from build123d import *

# Parameters (mm, degrees)
SKETCH_1_R               = 5
SKETCH_1_R_2             = 2.15
EXTRUDE_1_DEPTH          = 3
SKETCH_2_R               = 1.5
CUT_EXTRUDE_1_DEPTH      = 117.657618697
CUT_EXTRUDE_3_DEPTH      = 117.657618697
SKETCH_5_W               = 40
SKETCH_5_H               = 20
SKETCH_5_R               = 2.15
EXTRUDE_2_DEPTH          = 3
SKETCH_6_R               = 5
CUT_EXTRUDE_4_DEPTH      = 117.657618697
SKETCH_7_R               = 1.5
EXTRUDE_4_DEPTH          = 3
CUT_EXTRUDE_6_DEPTH      = 117.657618697
CUT_EXTRUDE_6_DEPTH_BACK = 117.657618697
SKETCH_9_R               = 1.6
CUT_EXTRUDE_7_DEPTH      = 117.657618697
SKETCH_10_W              = 79.9
SKETCH_10_H              = 10
SKETCH_10_R              = 1.6
EXTRUDE_5_DEPTH          = 3
FILLET_1_R               = 2.5


with BuildPart() as part:
    # ｽｹｯﾁ1 → ﾎﾞｽ - 押し出し1 (new body)
    with BuildSketch(Plane.XY):
        Polygon((10, 60), (0, 60), (0, 0), (100, 0), (100, 50), (100, 60), (50, 60), (50, 40), (10, 40), align=None)
        with Locations((20, 20)):
            Circle(SKETCH_1_R, mode=Mode.SUBTRACT)
        with Locations((5.25, 45)):
            Circle(SKETCH_1_R_2, mode=Mode.SUBTRACT)
        with Locations((5.25, 55)):
            Circle(SKETCH_1_R_2, mode=Mode.SUBTRACT)
        with Locations((54.75, 45)):
            Circle(SKETCH_1_R_2, mode=Mode.SUBTRACT)
        with Locations((54.75, 55)):
            Circle(SKETCH_1_R_2, mode=Mode.SUBTRACT)
    extrude(amount=EXTRUDE_1_DEPTH)

    # ｽｹｯﾁ2 → ｶｯﾄ - 押し出し1 (cut, through all)
    with BuildSketch(Plane.XY.offset(3)):
        with Locations((95, 35)):
            Circle(SKETCH_2_R)
    extrude(amount=-CUT_EXTRUDE_1_DEPTH, mode=Mode.SUBTRACT)

    # ｽｹｯﾁ4 → ｶｯﾄ - 押し出し3 (cut, through all)
    with BuildSketch(Plane.XY.offset(3)):
        with BuildLine():
            ThreePointArc((30.606601718, 9.393398282), (11.666446505, 7.527955815), (6.141807012, 25.740251485))
            ThreePointArc((6.141807012, 25.740251485), (5.992593584, 34.011854082), (1.731818145, 41.103219734))
            ThreePointArc((1.731818145, 41.103219734), (1.633577382, 41.194216579), (1.537689399, 41.287689399))
            ThreePointArc((1.537689399, 41.287689399), (0.399632454, 42.99091198), (0, 45))
            Line((0, 45), (0, 0))
            Line((0, 0), (100, 0))
            Line((100, 0), (100, 35))
            ThreePointArc((100, 35), (98.535533906, 31.464466094), (95, 30))
            ThreePointArc((95, 30), (93.906844507, 30.120962075), (92.866581158, 30.477995572))
            ThreePointArc((92.866581158, 30.477995572), (59.698938801, 28.658859349), (31.76111788, 10.689999666))
            ThreePointArc((31.76111788, 10.689999666), (31.202634234, 10.024981894), (30.606601718, 9.393398282))
        make_face()
    extrude(amount=-CUT_EXTRUDE_3_DEPTH, mode=Mode.SUBTRACT)

    # ｽｹｯﾁ5 → ﾎﾞｽ - 押し出し2 (add, through all)
    with BuildSketch(Plane.XY.offset(3)):
        with Locations((30, 50)):
            Rectangle(SKETCH_5_W, SKETCH_5_H)
        with Locations((5.25, 55)):
            Circle(SKETCH_5_R)
        with Locations((5.25, 45)):
            Circle(SKETCH_5_R)
        with Locations((54.75, 45)):
            Circle(SKETCH_5_R)
        with Locations((54.75, 55)):
            Circle(SKETCH_5_R)
    extrude(amount=-EXTRUDE_2_DEPTH)

    # ｽｹｯﾁ6 → ｶｯﾄ - 押し出し4 (cut, through all)
    with BuildSketch(Plane.XY.offset(3)):
        with Locations((20, 50)):
            Circle(SKETCH_6_R)
    extrude(amount=-CUT_EXTRUDE_4_DEPTH, mode=Mode.SUBTRACT)

    # ｽｹｯﾁ7 → ﾎﾞｽ - 押し出し4 (add, through all)
    # profile 1 of 2: a face of its own
    with BuildSketch(Plane.XY.offset(3)):
        with BuildLine():
            ThreePointArc((0, 45), (-1.007160055, 41.702552665), (-3.074339462, 38.943150628))
            ThreePointArc((-3.074339462, 38.943150628), (2.194117441, 39.492866419), (5, 35))
            ThreePointArc((5, 35), (2.338239569, 30.580425844), (-2.813054288, 30.866390733))
            ThreePointArc((-2.813054288, 30.866390733), (2.156646174, 25.048507639), (5.133931253, 18))
            ThreePointArc((5.133931253, 18), (5.125569714, 21.936833416), (6.141807012, 25.740251485))
            ThreePointArc((6.141807012, 25.740251485), (5.992593584, 34.011854082), (1.731818145, 41.103219734))
            ThreePointArc((1.731818145, 41.103219734), (0.4524509, 42.867859613), (0, 45))
        make_face()
    # profile 2 of 2: a face of its own
    with BuildSketch(Plane.XY.offset(3)):
        with BuildLine():
            ThreePointArc((-3.074339462, 38.943150628), (-3.301799792, 38.735793058), (-3.535533906, 38.535533906))
            ThreePointArc((-3.535533906, 38.535533906), (-5, 35), (-3.535533906, 31.464466094))
            ThreePointArc((-3.535533906, 31.464466094), (-3.171489153, 31.168816808), (-2.813054288, 30.866390733))
            ThreePointArc((-2.813054288, 30.866390733), (2.338239569, 30.580425844), (5, 35))
            ThreePointArc((5, 35), (2.194117441, 39.492866419), (-3.074339462, 38.943150628))
        make_face()
        with Locations((0, 35)):
            Circle(SKETCH_7_R, mode=Mode.SUBTRACT)
    extrude(amount=-EXTRUDE_4_DEPTH)

    # ｽｹｯﾁ9 → ｶｯﾄ - 押し出し6 (cut, two sides: drawn at the far end of the back side and taken through both)
    with BuildSketch(Plane.XY.offset(3).offset(-CUT_EXTRUDE_6_DEPTH_BACK)):
        with Locations((64.9, 55)):
            Circle(SKETCH_9_R)
    extrude(amount=CUT_EXTRUDE_6_DEPTH + CUT_EXTRUDE_6_DEPTH_BACK, mode=Mode.SUBTRACT)

    # ｽｹｯﾁ8 → ｶｯﾄ - 押し出し7 (cut, through all)
    with BuildSketch(Plane.XY.offset(3)):
        with BuildLine():
            ThreePointArc((95, 56.6), (93.4, 55), (95, 53.4))
            Line((95, 53.4), (95, 56.6))
        make_face()
        with BuildLine():
            Line((95, 56.6), (95, 53.4))
            ThreePointArc((95, 53.4), (96.13137085, 53.86862915), (96.6, 55))
            ThreePointArc((96.6, 55), (96.13137085, 56.13137085), (95, 56.6))
        make_face()
    extrude(amount=-CUT_EXTRUDE_7_DEPTH, mode=Mode.SUBTRACT)

    # ｽｹｯﾁ10 → ﾎﾞｽ - 押し出し5 (add, through all)
    with BuildSketch(Plane.XY.offset(3)):
        with Locations((39.95, 65)):
            Rectangle(SKETCH_10_W, SKETCH_10_H)
        with Locations((75.506601718, 65.606601718)):
            Circle(SKETCH_10_R, mode=Mode.SUBTRACT)
    extrude(amount=-EXTRUDE_5_DEPTH)

    # ﾌｨﾚｯﾄ1
    fillet_1_edges = [part.edges().sort_by_distance(p)[0] for p in [
        (0, 70, 1.5),
        (79.9, 70, 1.5),
        (79.9, 60, 1.5),
        (100, 60, 1.5),
    ]]
    fillet(fillet_1_edges, radius=FILLET_1_R)


solid = part.part
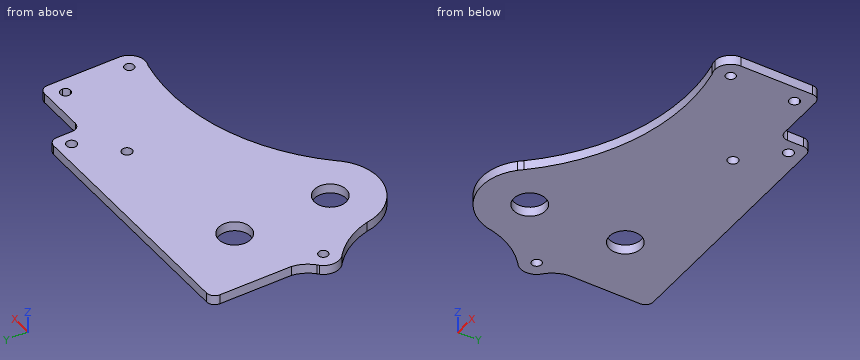
Input: part model. Units: mm. Frame: model coordinates. Coordinates: 2 decimals unless noted, no trailing zeros. Order: outer loops, then holes, each group sorted by start corner. A loop starts at its lowest first (then second) coordinate and runs counter-clockwise, first axis right, second up. Notation, with made-up numbers: M 3.25,-28 L 51.25,-28 A32 ccw 51.25,8 Z; hole C 11.5,9 d11. An arc over 180 degrees is marked long. Answer in a Markdown table with one row per item.
(1) Section query A-A, the plane y = 50. Output: boundary loops of the cut face in (x, z), plus the area to 3 significant figures.
Numbers:
| item | result |
|---|---|
| outline | M 0,0 L 15,0 L 15,3 L 0,3 Z; M 25,0 L 100,0 L 100,3 L 25,3 Z |
| area | 270 mm^2 |
(2) Contact query for flat-ended pins moving along their axis: pin 1 Ø1.5 at (y, z) = (14.5, 2.5) entering from -X; pin 2 Ø0.9 at (y, z) = (64, 2) entering from +X; pin 3 Ø1.5 at (y, z) = (59.5, 1) entering from -X. Output: stop coordinate, or through.
Numbers:
| item | result |
|---|---|
| pin 1 | stops at x = 5.77 |
| pin 2 | stops at x = 79.9 |
| pin 3 | stops at x = 0 |
(3) Material intervals for line 1 (Y direction, x = 20, z = 2.1); line 2 (Y direction, x = 95, z = 0.6); line 3 (X direction, y = 18.5, z = 0.2), sorted ascending. Write a range as [from, to].
Numbers:
| item | result |
|---|---|
| line 1 | y = [5, 15], [25, 45], [55, 70] |
| line 2 | y = [30, 33.5], [36.5, 53.4], [56.6, 60] |
| line 3 | x = [5, 15.23], [24.77, 40.3] |
(4) Section query B-B, the plane x = 20. Output: boundary loops of the cut face in (y, z), plus the area to 3 significant figures.
Numbers:
| item | result |
|---|---|
| outline | M 5,0 L 15,0 L 15,3 L 5,3 Z; M 25,0 L 45,0 L 45,3 L 25,3 Z; M 55,0 L 70,0 L 70,3 L 55,3 Z |
| area | 135 mm^2 |
(5) Section query C-C, the plane x = 64.9. Output: boundary loops of the cut face in (y, z), plus the area to 3 significant figures.
Numbers:
| item | result |
|---|---|
| outline | M 30.11,0 L 53.4,0 L 53.4,3 L 30.11,3 Z; M 56.6,0 L 70,0 L 70,3 L 56.6,3 Z |
| area | 110 mm^2 |
(6) Section query D-D, the plane z = 1.2. Output: boundary loops of the cut face in (x, y).
Numbers:
| item | result |
|---|---|
| outline | M -3.54,31.46 A25 cw 5.13,18 A15 ccw 31.76,10.69 A65 cw 92.87,30.48 A5 ccw 100,35 L 100,57.5 A2.5 ccw 97.5,60 L 82.4,60 A2.5 cw 79.9,62.5 L 79.9,67.5 A2.5 ccw 77.4,70 L 2.5,70 A2.5 ccw 0,67.5 L 0,45 A10 cw -3.54,38.54 A5 ccw Z; hole C 0,35 d3; hole C 20,20 d10; hole C 20,50 d10; hole C 64.9,55 d3.2; hole C 75.51,65.61 d3.2; hole C 95,55 d3.2; hole C 95,35 d3 |
